from build123d import *

# Parameters (mm, degrees)
F0_W     = 70
F0_H     = 470
F1_DEPTH = 685
F0_W_2   = 930
F0_H_2   = 900
F2_DEPTH = 525
F3_T     = 2.5
F4_DEPTH = 685
F5_DEPTH = 75


with BuildPart() as f1:
    # F0 (on Right) → F1 (new body, symmetric)
    with BuildSketch(Plane.YZ):
        Polygon((0, -725), (0, 0), (-880, 0), (-880, -900), (-880, -1010), (-860, -1010), (-860, -678.4179210663), (-310, -678.4179210663), (-310, -1010), (-380, -1010), (-380, -1195), (-70, -1195), (-70, -725), align=None)
        with Locations((-35, -960)):
            Rectangle(F0_W, F0_H)
        Polygon((-860, -678.4179210663), (-860, -1010), (-380, -1010), (-310, -1010), (-310, -678.4179210663), align=None)
    extrude(amount=F1_DEPTH, both=True)

    # F0 (on Right) → F2 (join, symmetric)
    with BuildSketch(Plane.YZ):
        with Locations((-1345, -450)):
            Rectangle(F0_W_2, F0_H_2)
    extrude(amount=F2_DEPTH, both=True)

    # F3
    f3_openings = [f1.faces().sort_by_distance(p)[0] for p in [
        (0, -1810, -450),
    ]]
    offset(amount=F3_T, openings=f3_openings, kind=Kind.INTERSECTION)

    # F0 (on Right) → F4 (join, symmetric)
    with BuildSketch(Plane.YZ):
        Polygon((-860, -678.4179210663), (-860, -1010), (-380, -1010), (-310, -1010), (-310, -678.4179210663), align=None)
    extrude(amount=F4_DEPTH, both=True)

    # F0 (on Right) → F5 (join, symmetric)
    with BuildSketch(Plane.YZ):
        with Locations((-35, -960)):
            Rectangle(F0_W, F0_H)
    extrude(amount=F5_DEPTH, both=True)


solid = f1.part
For this review, take the finished solid that the model builds, in its own axes (mm). A direction names the side the tool comes from. Coordinates: 2 decimals unless noted, no trailing zeros. Loops run counter-clockwise (first coordinate to the right, second up) from the corner with the lowest first, then second, coordinate; pieces in that order, holes last. Notation, with made-up numbers: (26, 55.5) - (33, 55.5) arc R9 ccw to (33, 59.5) - close; hole circle Ø1 at (-11, 30.25). An arc over 180 degrees is marked (long way). Return JSON: item names as keys, results as strings.
Item 1: Take a section at A-A (y = -424). Give the boundary of the cut face in (x, z), then the cut area to 3 significant figures.
Determined:
{"outline": "(-687.5, -1012.5) - (687.5, -1012.5) - (687.5, 2.5) - (-687.5, 2.5) - close; hole (-685, -678.42) - (685, -678.42) - (685, 0) - (-685, 0) - close", "area": "466,000 mm2"}
Item 2: Take a section at B-B (x = -555.5). Give the boundary of the cut face in (y, z), then the cut area to 3 significant figures.
Determined:
{"outline": "(-882.5, -1012.5) - (-382.5, -1012.5) - (-382.5, -1197.5) - (2.5, -1197.5) - (2.5, 2.5) - (-882.5, 2.5) - close; hole (-880, -1010) - (-860, -1010) - (-860, -678.42) - (-310, -678.42) - (-310, -1010) - (-380, -1010) - (-380, -1195) - (0, -1195) - (0, 0) - (-880, 0) - close", "area": "193,000 mm2"}
Item 3: For faces 1 (the flat face through (525, -1352, -444)), 2 (the flat face through (-527.5, -1353, -444)), 3 (the flat face through (10, -310, -847)), 4 (the flat face through (10, -382.5, -1104)), list the 3-axis set-ups (+Z, -Z, +X, -X, +Y, -Y) from which the entire face can be reached by the end or side of a thin tool; tool diameter is ignored.
Determined:
{"face 1": "-Y", "face 2": "+Z, -Z, -X, -Y", "face 3": "none", "face 4": "-Z, +X, -X, -Y"}
Item 4: Take a section at C-C (z = -374). Give the boundary of the cut face in (x, y).
Determined:
{"outline": "(-687.5, -882.5) - (-527.5, -882.5) - (-527.5, -1810) - (-525, -1810) - (-525, -880) - (-685, -880) - (-685, 0) - (685, 0) - (685, -880) - (525, -880) - (525, -1810) - (527.5, -1810) - (527.5, -882.5) - (687.5, -882.5) - (687.5, 2.5) - (-687.5, 2.5) - close"}
Item 5: Mouldability with a two-part tool opening along Z and no side actions: class faces 5 (the flat face through (-685, -348, -456)), 6 (the flat face through (687.5, -446, -589)), 7 (the flat face through (10, -891, 2.5)) as pulls with the +Z half, pulls with the -Z half, needs draft (parallel to the pull), parting line crosses it, or undercut.
Determined:
{"face 5": "undercut", "face 6": "needs draft", "face 7": "pulls with the +Z half"}
Item 6: For line 1 (Y direction, x = 542.5, z = -831.5); line 2 (Z direction, x = -270, y = -326); line 3 (X direction, y = -1441, z = -887), list the stretches that pass through material, from the lowest coordinate up.
Determined:
{"line 1": "y = -882.5 to -880, -860 to -310, 0 to 2.5", "line 2": "z = -1197.5 to -1195, -1010 to -678.42, 0 to 2.5", "line 3": "x = -527.5 to -525, 525 to 527.5"}
Item 7: Insertion check: pin 1 (12 mm diameter, centred on x = -224, y = -1545, fed in from -Z). The pin has a flat end and moves straight along its axis. Give the tip position at first contact, or say it passes through.
Determined:
{"pin 1": "stops at z = -902.5"}
Item 8: Take a section at D-D (x = 203). Give the boundary of the cut face in (y, z), then the cut area to 3 significant figures.
Determined:
{"outline": "(-1810, -902.5) - (-882.5, -902.5) - (-882.5, -1012.5) - (-382.5, -1012.5) - (-382.5, -1197.5) - (2.5, -1197.5) - (2.5, 2.5) - (-1810, 2.5) - (-1810, 0) - (0, 0) - (0, -1195) - (-380, -1195) - (-380, -1010) - (-310, -1010) - (-310, -678.42) - (-860, -678.42) - (-860, -1010) - (-880, -1010) - (-880, -900) - (-1810, -900) - close", "area": "195,000 mm2"}
